Design review of the part built by this model. Coordinates are the model's own, in mm. Coordinates: 2 decimals unless noted, no trailing zeros. Write each loop counter-clockwise with the first axis right and the second up, starting at its lowest first coordinate (ties: lowest second). Pieces come first, ordered by that corner, then holes. Notation, with made-up numbers: M 65,83 L 84,83 A15 cw 84,105 Z; hole C 81,15 d10. An arc over 180 degrees is marked long. Write each question's results on one line, items separated by ' | '. Start each with the question number.
```python
from build123d import *

# Parameters (mm, degrees)
SKETCH1_W              = 323.85
SKETCH1_H              = 127
BOSS_EXTRUDE1_DEPTH    = 3.175
CUT_EXTRUDE1_DEPTH     = 4.175
SKETCH3_R              = 6.35
CUT_EXTRUDE2_DEPTH     = 58.15
F_10_CLEARANCE_HOLE1_D = 5.1054


with BuildPart() as part:
    # Sketch1 → Boss-Extrude1 (new body)
    with BuildSketch(Plane(origin=(0, 0, 0), x_dir=(1, 0, 0), z_dir=(0, 1, 0))):
        with Locations((161.925, 63.5)):
            Rectangle(SKETCH1_W, SKETCH1_H)
    extrude(amount=BOSS_EXTRUDE1_DEPTH)

    # Sketch2 → Cut-Extrude1 (cut, through all)
    with BuildSketch(Plane(origin=(0, 3.175, 0), x_dir=(1, 0, 0), z_dir=(0, 1, 0))):
        with BuildLine():
            Line((25.4, 127), (25.4, 111.125))
            ThreePointArc((25.4, 111.125), (31.75, 104.775), (38.1, 111.125))
            Line((38.1, 111.125), (38.1, 127))
            Line((38.1, 127), (25.4, 127))
        make_face()
    extrude(amount=-CUT_EXTRUDE1_DEPTH, mode=Mode.SUBTRACT)

    # Sketch3 → Cut-Extrude2 (cut, through all)
    with BuildSketch(Plane(origin=(0, -53.975, 0), x_dir=(-1, 0, 0), z_dir=(0, -1, 0))):
        with Locations((-285.75, 112.649)):
            Circle(SKETCH3_R)
    extrude(amount=-CUT_EXTRUDE2_DEPTH, mode=Mode.SUBTRACT)

    # #10 Clearance Hole1 (through all)
    with Locations(Plane(origin=(0, 3.175, 0), x_dir=(1, 0, 0), z_dir=(0, 1, 0))):
        with Locations((315.9125, 56.25), (315.9125, 70.75), (7.9375, 56.25), (7.9375, 70.75)):
            Hole(F_10_CLEARANCE_HOLE1_D / 2)


solid = part.part
```
Item 1: We need section A-A on x = 285.75. State the section outline as (y, z) points (3 decimals).
Item 2: Insertion check: pin 1 Ø1 at (x, z) = (111.5, -66.5) entering from -Y. The pin has a flat end and moves straight along its axis. Give the tip position at first contact, or say it passes through.
Item 3: We need section B-B on x = 31.75. State the section outline as (y, z) points (3 decimals).
Item 4: Draft analysis for pull direction X (two halves, no side actions). For faces 1 (the cylindrical face through (292.094, 1.565, -112.928)), 2 (the flat face through (160, 3.175, -64)), state which applies: released by +X, released by -X, zero draft, split by the parting line, or undercut.
Item 5: Wall thickness on L1, parallel to X at y = 2, z = -56.25; L2, parallel to Z at x = 285.75, y = 1.8; L3, parallel to X at y = 0.25, z = -116.5: over which ranges is each line inside the solid? List them lowest first.
Answer:
1) outline: M 0,-127 L 3.175,-127 L 3.175,-118.999 L 0,-118.999 Z; M 0,-106.299 L 3.175,-106.299 L 3.175,0 L 0,0 Z
2) pin 1: stops at y = 0
3) outline: M 0,-104.775 L 3.175,-104.775 L 3.175,0 L 0,0 Z
4) face 1: undercut | face 2: zero draft
5) L1: x = 0 to 5.38, 10.49 to 313.36, 318.47 to 323.85 | L2: z = -127 to -119, -106.3 to 0 | L3: x = 0 to 25.4, 38.1 to 280.7, 290.8 to 323.85
